Design review of the part built by this model. Coordinates are the model's own, in mm. A direction names the side the tool comes from. Coordinates: 2 decimals unless noted, no trailing zeros. Loops run counter-clockwise (first coordinate to the right, second up) from the corner with the lowest first, then second, coordinate; pieces in that order, holes last. Notation, with made-up numbers: (57, -37.5) - (90, -37.5) arc R20 ccw to (90, -17.5) - close; hole circle Ø9 at (3.25, -30). An arc over 180 degrees is marked (long way). Answer in a Markdown table with one row per item. Add a question column.
(1) For faces 1 (the face through (22, 25, 296)), 2 (the face through (2, 23, 600)), 3 (the face through (1.521, 23.348, 567.746)), list the 3-axis set-ups (+Z, -Z, +X, -X, +Y, -Y) from which the entire face can be reached by the end or side of a thin tool; tool diameter is ignored.
(2) To check wall thickness, follow L1, parallel to Z at x = 2.05, y = 25; L2, parallel to Z at x = 12.5, y = 1.1; L3, parallel to Z at x = 2.75, y = 24. State the ranges of each line that lie inside material, in increasing order. Write a range as [from, to].
(3) We need section A-A, the plane z = 474.5. Write out the cut boundary in (x, y).
(4) We need section B-B, the plane y = 11. Write out the cut boundary in (x, z).
(5) Clearance check with flat-ended pins moving along their axes: pin 1 (6 mm diameter, centred on x = 8.5, y = 26, fed in from +Z); pin 2 (17.5 mm diameter, centred on y = 25, z = 37.5, fed in from +X); pin 3 (4.5 mm diameter, centred on x = 12.5, z = 300, fed in from -Y). State where each tip first meets the part, or that it passes through.
(6) The part is to be moulded in two halves that separate along Y. For faces 4 (the face through (13, 50, 296)), 5 (the face through (13, 3, 296)), 6 (the face through (2, 23, 0)), say which applies: released by +Y, released by -Y, zero draft, split by the parting line, or undercut.
Autodesk Inventor part; units mm, degrees
ref_plane "YZ Plane" through (0, 0, 0) normal (1, 0, 0) x (0, 1, 0)
ref_plane "XZ Plane" through (0, 0, 0) normal (0, 1, 0) x (-1, 0, 0)
ref_plane "XY Plane" through (0, 0, 0) normal (0, 0, 1) x (1, 0, 0)
sketch "Sketch1" plane through (0, 0, 0) normal (0, 0, 1) x (1, 0, 0)
  line L0 (0, 0) -> (25, 0)
  line L1 (25, 0) -> (25, 50)
  line L2 (25, 50) -> (0, 50)
  line L3 (0, 50) -> (0, 0)
  line L4 (22, 47) -> (22, 3)
  line L5 (22, 3) -> (3, 3)
  line L6 (3, 3) -> (3, 47)
  line L7 (3, 47) -> (22, 47)
  dimension "d0" = 25
  dimension "d1" = 50
  dimension "d2" = 3
extrude "Extrusion1" add sketch "Sketch1" along normal blind 600
sketch "Sketch2" plane through (0, 0, 0) normal (1, 0, 0) x (0, 0, -1)
  line L0 (0, 0) -> (-600, 0)
  line L1 (-600, 0) -> (-600, 50)
  point P0 (-562.5, 25)
  point P1 (-37.5, 25)
  dimension "d5" = 25
  dimension "d6" = 37.5
  dimension "d7" = 37.5
hole "Hole1" at (0, 25, 562.5) at (0, 25, 37.5) direction (1, 0, 0) diameter 6 end through all counterbore diameter 11 counterbore depth 5
sketch "Sketch3" plane through (0, 0, 0) normal (0, -1, 0) x (1, 0, 0)
  line L0 (0, 0) -> (25, 0)
  line L1 (0, 0) -> (0, 600)
  point P0 (12.5, 100)
  point P1 (12.5, 200)
  point P2 (12.5, 300)
  point P3 (12.5, 400)
  point P4 (12.5, 500)
  dimension "d15" = 100
  dimension "d16" = 12.5
  dimension "d19" = 100
hole "Hole2" at (12.5, 0, 100) at (12.5, 0, 200) at (12.5, 0, 300) at (12.5, 0, 400) at (12.5, 0, 500) direction (0, 1, 0) diameter 5 depth 8 tip angle 118
properties part number "Front Bar"
Responses:
| question | item | result |
|---|---|---|
| 1 | face 1 | +Z, -Z |
| 1 | face 2 | +Z, +X, -X, +Y, -Y |
| 1 | face 3 | -X |
| 2 | L1 | z = [0, 32], [43, 557], [568, 600] |
| 2 | L2 | z = [0, 97.5], [102.5, 197.5], [202.5, 297.5], [302.5, 397.5], [402.5, 497.5], [502.5, 600] |
| 2 | L3 | z = [0, 32.09], [42.91, 557.09], [567.91, 600] |
| 3 | outline | (0, 0) - (25, 0) - (25, 50) - (0, 50) - close; hole (3, 3) - (22, 3) - (22, 47) - (3, 47) - close |
| 4 | outline | (0, 0) - (3, 0) - (3, 600) - (0, 600) - close; (22, 0) - (25, 0) - (25, 600) - (22, 600) - close |
| 5 | pin 1 | passes through |
| 5 | pin 2 | stops at x = 25 |
| 5 | pin 3 | stops at y = 47 |
| 6 | face 4 | released by +Y |
| 6 | face 5 | undercut |
| 6 | face 6 | zero draft |
